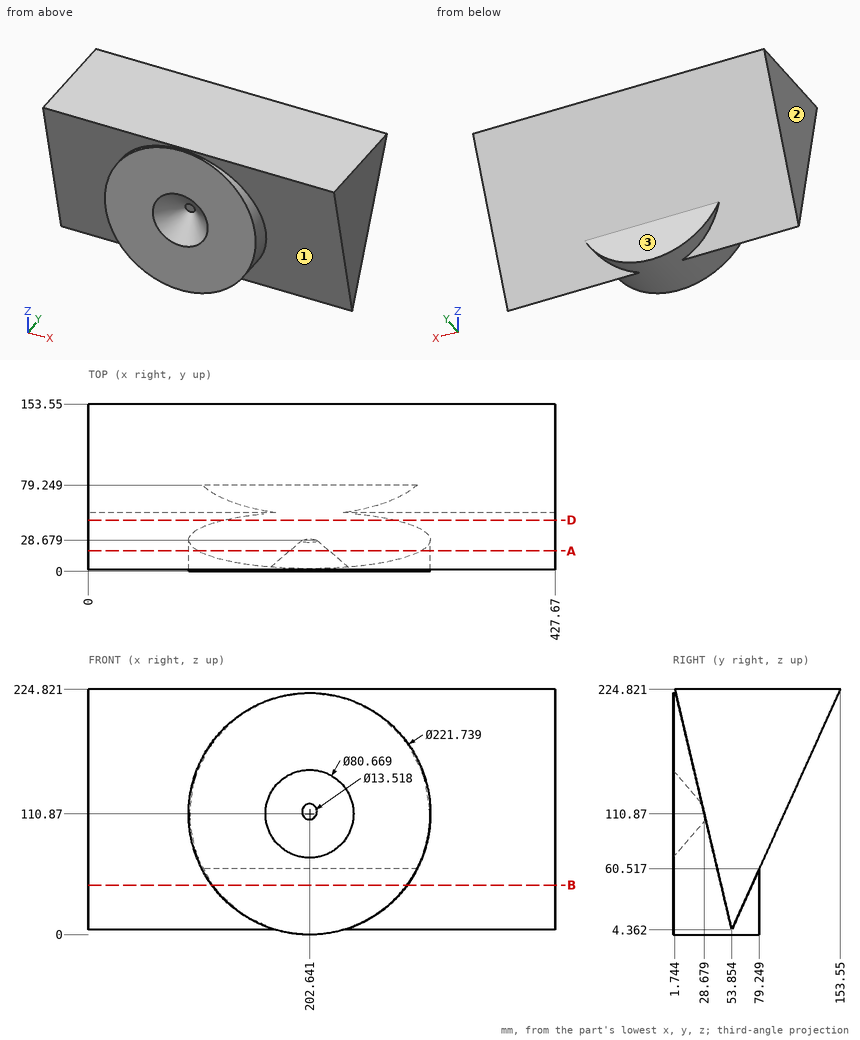
The drawing under review shows one solid part. Ordinate dimensions are in mm from its lowest x, y, z. A direction names the side the tool comes from. Give positions to 0.01 mm unless a question says otherwise; leave off trailing zeros. Loops run counter-clockwise (first coordinate to the right, second up) from the corner with the lowest first, then second, coordinate; pieces in that order, holes last. Notation, with made-up numbers: M 50,5.5 L 68,5.5 A16 ccw 68,15.5 Z; hole C 78,47.25 d5. An arc over 180 degrees is marked long. One line per question, with ' | ' between items. Start each with the question number.
1. Add section A-A (y = 19). Write out the cut boundary in (x, z), plus the area to 3 significant figures.
2. For the marked faces 1, 2 and 3, list the 3-axis set-ups (+Z, -Z, +X, -X, +Y, -Y) from which the entire face can be reached by the end or side of a thin tool; tool diameter is ignored.
3. Add section D-D (y = 47). Write out the cut boundary in (x, z), plus the area to 3 significant figures.
4. Insertion check: P1, Ø1.5, axis at x = 334.5, z = 160.5, coming from the -Y side; P2, Ø5, axis at x = 378, z = 105, coming from the -Y side (1 decimal); P3, Ø1, axis at x = 372, z = 95.5, coming from the +Y side (1 decimal). Each pin has a flat end and moves straight along its axis. Give the tip position at first contact, or say it passes through.
5. To check wall thickness, follow L1, parallel to Y at x = 265, z = 53.5; L2, parallel to Y at x = 373, z = 192; L3, parallel to Z at x = 67.5, y = 96 (1 decimal). State the ranges of each line that lie inside material, in increasing order.
6. Add section B-B (z = 45.5). Write out the cut boundary in (x, y), plus the area to 3 significant figures.
Worked out:
1) outline: M 0,151.82 L 99.61,151.82 A110.87 ccw long 305.67,151.82 L 427.67,151.82 L 427.67,224.82 L 0,224.82 Z; hole C 202.64,110.87 d36.18 | area: 58,400 mm²
2) face 1: -Y | face 2: +Z, -Z, -X, +Y, -Y | face 3: -Z, +X, -X, +Y
3) outline: M 0,33.36 L 123.37,33.36 A110.87 ccw 281.91,33.36 L 427.67,33.36 L 427.67,224.82 L 0,224.82 Z | area: 85,500 mm²
4) P1: stops at y = 16.77 | P2: stops at y = 29.5 | P3: stops at y = 95.3
5) L1: y = 0 to 79.25 | L2: y = 9.5 to 138.71 | L3: z = 97.6 to 224.8
6) outline: M 0,44.13 L 113.09,44.13 L 113.09,0 L 292.19,0 L 292.19,44.13 L 427.67,44.13 L 427.67,72.46 L 292.19,72.46 L 292.19,79.25 L 113.09,79.25 L 113.09,72.46 L 0,72.46 Z | area: 21,200 mm²
